Design review of the part built by this model. Coordinates are the model's own, in mm. Coordinates: 2 decimals unless noted, no trailing zeros. Write each loop counter-clockwise with the first axis right and the second up, starting at its lowest first coordinate (ties: lowest second). Pieces come first, ordered by that corner, then holes.
Q1. Insertion check: pin 1 (3 mm diameter, centred on x = -22, z = 1.5, fed in from -Y). The pin has a flat end and moves straight along its axis. Give the tip position at first contact, or say it passes through.
Q2. For probe 1 along Y at (x, z) = (-46.5, 14); probe 2 along X at (y, z) = (-111, 13); probe 3 along Y at (x, z) = (-59.5, 11.75), list the stretches that pass through material, from the lowest coordinate up.
Q3. Take a section at A-A (z = 12.75). Give the boundary of the cut face in (x, y), and give its area (3 significant figures).
```python
from build123d import *

# Parameters (mm, degrees)
ESQUISSE1_W        = 70
ESQUISSE1_H        = 140
BOSS_EXTRU_1_DEPTH = 15
CONG_1_R           = 4
CONG_2_R           = 4
CONG_3_R           = 4


with BuildPart() as part:
    # Esquisse1 → Boss.-Extru.1 (new body)
    with BuildSketch(Plane.XY):
        with Locations((-35, -70)):
            Rectangle(ESQUISSE1_W, ESQUISSE1_H)
    extrude(amount=BOSS_EXTRU_1_DEPTH)

    # Congé1
    cong_1_edges = [part.edges().sort_by_distance(p)[0] for p in [
        (0, -140, 7.5),
        (-70, -140, 7.5),
        (-70, 0, 7.5),
        (0, 0, 7.5),
    ]]
    fillet(cong_1_edges, radius=CONG_1_R)

    # Congé2
    cong_2_edges = [part.edges().sort_by_distance(p)[0] for p in [
        (0, -70, 15),
        (-35, -140, 15),
        (-35, 0, 15),
        (-70, -70, 15),
        (-1.171572875, -1.171572875, 15),
        (-68.828427125, -1.171572875, 15),
        (-68.828427125, -138.828427125, 15),
        (-1.171572875, -138.828427125, 15),
    ]]
    fillet(cong_2_edges, radius=CONG_2_R)

    # Congé3
    cong_3_edges = [part.edges().sort_by_distance(p)[0] for p in [
        (0, -70, 0),
        (-35, -140, 0),
        (-70, -70, 0),
        (-35, 0, 0),
        (-1.171572875, -1.171572875, 0),
        (-68.828427125, -1.171572875, 0),
        (-68.828427125, -138.828427125, 0),
        (-1.171572875, -138.828427125, 0),
    ]]
    fillet(cong_3_edges, radius=CONG_3_R)


solid = part.part
```
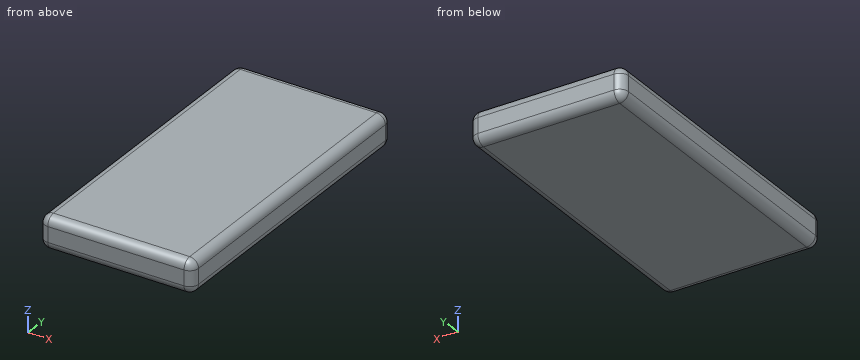
Response:
1. pin 1: stops at y = -139.87
2. probe 1: y = -138.65 to -1.35
2. probe 2: x = -69.46 to -0.54
2. probe 3: y = -139.93 to -0.07
3. outline: (-69.6, -136) arc R3.6 ccw to (-66, -139.6) - (-4, -139.6) arc R3.6 ccw to (-0.4, -136) - (-0.4, -4) arc R3.6 ccw to (-4, -0.4) - (-66, -0.4) arc R3.6 ccw to (-69.6, -4) - close
3. area: 9,620 mm2
